from build123d import *

# Parameters (mm, degrees)
F0_R     = 33
F1_DEPTH = 20
F2_T     = -2
F3_DEPTH = 102
F4_W     = 23.5
F4_H     = 23.5
F5_DEPTH = 12.5
F6_W     = 13
F6_H     = 3
F6_H_2   = 2.9999976491
F7_DEPTH = 7


# Not quite as in the source:
# - an extrude ends at something that could not be found from the text; its depth is read off the source's solid


with BuildPart() as f1:
    # F0 (on Top) → F1 (new body)
    with BuildSketch(Plane.XY):
        Circle(F0_R)
    extrude(amount=F1_DEPTH)

    # F2
    f2_openings = [f1.faces().sort_by_distance(p)[0] for p in [
        (0, 0, 20),
    ]]
    offset(amount=F2_T, openings=f2_openings)

    # F0 (on Top) → F3 (cut, through all)
    with BuildSketch(Plane.XY):
        Circle(F0_R)
    extrude(amount=-F3_DEPTH, mode=Mode.SUBTRACT)

    # F4 (on face) → F5 (cut, symmetric)
    with BuildSketch(Plane.XY):
        Rectangle(F4_W, F4_H)
    extrude(amount=F5_DEPTH, both=True, mode=Mode.SUBTRACT)

    # F6 (on Top) → F7 (join)
    with BuildSketch(Plane.XY):
        with Locations((0, 14.5980315283)):
            Rectangle(F6_W, F6_H)
        with Locations((0, -14.5859429613)):
            Rectangle(F6_W, F6_H_2)
    extrude(amount=F7_DEPTH)


solid = f1.part
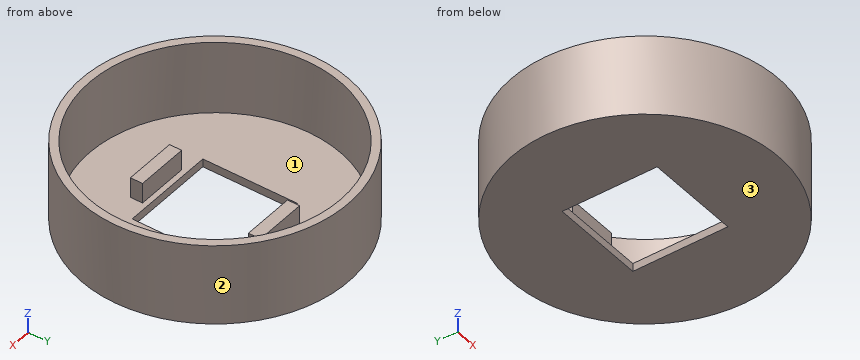
The model under review builds one solid part; all positions refer to its coordinate system, in mm. Face numbers are marked on the shaded views. Coordinates: 2 decimals unless noted, no trailing zeros. Loops run counter-clockwise (first coordinate to the right, second up) from the corner with the lowest first, then second, coordinate; pieces in that order, holes last. Notation, with made-up numbers: (-38, 54) -> (-11, 54) arc R27 ccw to (-11, 89) -> close; hole circle Ø10 at (63.25, 6.25). An arc over 180 degrees is marked (long way). Use a Markdown table: item, result. Add a question column.
1. Draft analysis for pull direction X (two halves, no side actions). For the marked faces 1, 2 and 3, state which applies: pulls with the +X half, pulls with the -X half, needs draft (parallel to the pull), parting line crosses it, or undercut.
2. Add section A-A on z = 3. Write out the cut boundary in (x, y).
3. Clearance check with flat-ended pins moving along their axes: pin 1 Ø4 at (x, z) = (11.5, 4) entering from -Y; pin 2 Ø2.5 at (y, z) = (-14, 5) entering from +X; pin 3 Ø1 at (y, z) = (-1, 0.5) entering from +X. State where each tip first meets the part, or that it passes through.
4. Add section B-B on x = 0. Write out the cut boundary in (y, z), plus the area to 3 significant figures.
5. Add section D-D on z = 15.75. Write out the cut boundary in (x, y), plus the area to 3 significant figures.
6. Add section C-C on y = 0. Write out the cut boundary in (x, z), plus the area to 3 significant figures.
7. To check wall thickness, follow line 1 (Y direction, x = 0, z = 6.5); line 2 (Y direction, x = 0, z = 13); line 3 (Z direction, x = -19.5, y = 10). State the ranges of each line that lie inside material, in increasing order.
Returned:
| question | item | result |
|---|---|---|
| 1 | face 1 | undercut |
| 1 | face 2 | parting line crosses it |
| 1 | face 3 | needs draft |
| 2 | outline | circle Ø66 at (0, 0); (-6.5, -16.09) -> (6.5, -16.09) -> (6.5, -13.09) -> (-6.5, -13.09) -> close; (-6.5, 13.1) -> (6.5, 13.1) -> (6.5, 16.1) -> (-6.5, 16.1) -> close; hole circle Ø62 at (0, 0) |
| 3 | pin 1 | stops at y = -31.6 |
| 3 | pin 2 | stops at x = 30.44 |
| 3 | pin 3 | stops at x = 33 |
| 4 | outline | (-33, 0) -> (-11.75, 0) -> (-11.75, 2) -> (-13.09, 2) -> (-13.09, 7) -> (-16.09, 7) -> (-16.09, 2) -> (-31, 2) -> (-31, 20) -> (-33, 20) -> close; (11.75, 0) -> (33, 0) -> (33, 20) -> (31, 20) -> (31, 2) -> (16.1, 2) -> (16.1, 7) -> (13.1, 7) -> (13.1, 2) -> (11.75, 2) -> close |
| 4 | area | 187 mm² |
| 5 | outline | circle Ø66 at (0, 0); hole circle Ø62 at (0, 0) |
| 5 | area | 402 mm² |
| 6 | outline | (-33, 0) -> (-11.75, 0) -> (-11.75, 2) -> (-31, 2) -> (-31, 20) -> (-33, 20) -> close; (11.75, 0) -> (33, 0) -> (33, 20) -> (31, 20) -> (31, 2) -> (11.75, 2) -> close |
| 6 | area | 157 mm² |
| 7 | line 1 | y = -33 to -31, -16.09 to -13.09, 13.1 to 16.1, 31 to 33 |
| 7 | line 2 | y = -33 to -31, 31 to 33 |
| 7 | line 3 | z = 0 to 2 |
